Geometry check sheet. Reference: the model listing, model coordinates, mm. Face numbers are marked on the shaded views. A direction names the side the tool comes from. Coordinates: 2 decimals unless noted, no trailing zeros. Order: outer loops, then holes, each group sorted by start corner. A loop starts at its lowest first (then second) coordinate and runs counter-clockwise, first axis right, second up. Notation, with made-up numbers: (17.25, 36.25) - (43.25, 36.25) arc R26 ccw to (43.25, 75.25) - close; hole circle Ø8 at (-19, -29.75). An arc over 180 degrees is marked (long way). Return JSON: item names as keys, results as strings. Group by question number.
Item 1: Section check C-C on y = 19.5. Enter the section's corners in (x, z).
Item 2: Section check B-B on y = 10. Enter the section's corners in (x, z), then the cut area to 3 significant figures.
Item 3: Draft check along Y on the marked faces 3, 4 and 5. Enter one of: pulls with the +Y half, pulls with the -Y half, needs draft (parallel to the pull), parting line crosses it, or undercut.
Item 4: Tool access check on the marked faces 1 and 2. Record the directions out of +Z, -Z, +X, -X, +Y, -Y that give a thin tool (end or side, any length) a straight path to the whole face; none if there is none.
Item 5: Section check A-A on y = -18. Enter the section's corners in (x, z).
Item 6: Scan lines: probe 1 along Y at (x, z) = (-1.5, 2.25); probe 2 along Y at (x, z) = (-2, 2.5); probe 3 along Z at (x, y) = (0, -20.5). Record each from-to range of solid material in increasing order.
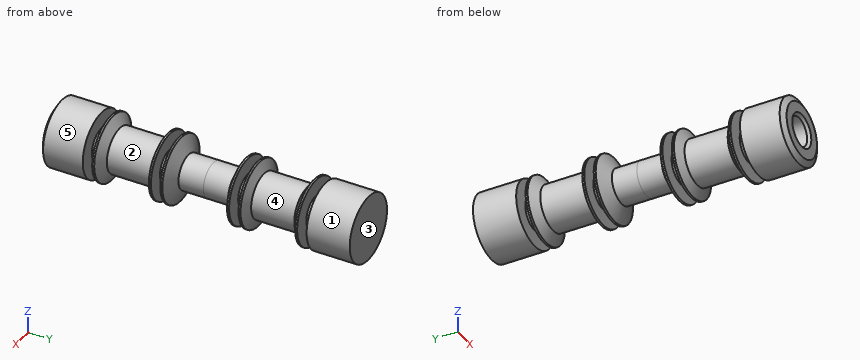
from build123d import *

# Parameters (mm, degrees)
MIDBODYS_R                           = 2.6
MIDBODY_DEPTH                        = 3.7
MIDORINGBODYS_R                      = 2.5
MIDORINGBODY_DEPTH                   = 1.4
EXTENDEDMIDBODYS_R                   = 3.35
EXTENDEDMIDBODY_DEPTH                = 6.4
ENDORINGBODYS_R                      = 2.5
ENDORINGBODY_DEPTH                   = 1.4
ENDBODY_START                        = 6.4
ENDBODYS_R                           = 4.9
ENDBODY_DEPTH                        = 6.4
F_4_2_4_2_DIAMETER_HOLE1_D           = 4.2
F_4_2_4_2_DIAMETER_HOLE1_DEPTH       = 9.4
F_4_2_4_2_DIAMETER_HOLE1_CSINK_D     = 5
F_4_2_4_2_DIAMETER_HOLE1_CSINK_ANGLE = 90
F_4_2_4_2_DIAMETER_HOLE1_TIP         = 1.2618073
CHAMFERS_OUTSIDE_W                   = 186.02
CHAMFERS_OUTSIDE_H                   = 186.02
CHAMFERS_OUTSIDE_R                   = 4
CHAMFER_2_DEPTH                      = 47.519028365
CHAMFER_2_DRAFT                      = -60


with BuildPart() as part:
    # MidBodyS → MidBody (new body)
    with BuildSketch(Plane(origin=(0, 0, 0), x_dir=(1, 0, 0), z_dir=(0, 1, 0))):
        with Locations(Location((0, 0, 0), (0, 0, 270))):
            Circle(MIDBODYS_R)
    midbody = extrude(amount=MIDBODY_DEPTH)

    # MidORingBaseS → MidORingBase (revolve)
    with BuildSketch(Plane.XY, mode=Mode.PRIVATE) as midoringbase_sk:
        Polygon((2.6, 3.7), (4.9, 4.8), (4.9, 5.1), (0, 5.1), (0, 3.7), align=None)
    midoringbase = revolve(midoringbase_sk.sketch.rotate(Axis((0, 5.1, 0), (0, -1, 0)), 180), axis=Axis((0, 5.1, 0), (0, -1, 0)))

    # MidORingBodyS → MidORingBody (add)
    with BuildSketch(Plane(origin=(0, 5.1, 0), x_dir=(1, 0, 0), z_dir=(0, 1, 0))):
        with Locations(Location((0, 0, 0), (0, 0, 180))):
            Circle(MIDORINGBODYS_R)
    midoringbody = extrude(amount=MIDORINGBODY_DEPTH)

    # MidORingTopBaseS → MidORingTopBase (revolve)
    with BuildSketch(Plane.XY, mode=Mode.PRIVATE) as midoringtopbase_sk:
        Polygon((0, 6.5), (4.9, 6.5), (4.9, 6.8), (3.35, 7.5), (0, 7.5), align=None)
    midoringtopbase = revolve(midoringtopbase_sk.sketch.rotate(Axis((0, 6.5, 0), (0, 1, 0)), 90), axis=Axis((0, 6.5, 0), (0, 1, 0)))

    # ExtendedMidBodyS → ExtendedMidBody (add)
    with BuildSketch(Plane(origin=(0, 7.5, 0), x_dir=(1, 0, 0), z_dir=(0, 1, 0))):
        with Locations(Location((0, 0, 0), (0, 0, 180))):
            Circle(EXTENDEDMIDBODYS_R)
    extendedmidbody = extrude(amount=EXTENDEDMIDBODY_DEPTH)

    # EndORingBaseS → EndORingBase (revolve)
    with BuildSketch(Plane.XY, mode=Mode.PRIVATE) as endoringbase_sk:
        Polygon((0, 15.2), (4.9, 15.2), (4.9, 14.9), (3.35, 13.9), (0, 13.9), align=None)
    endoringbase = revolve(endoringbase_sk.sketch.rotate(Axis((0, 13.9, 0), (0, 1, 0)), 90), axis=Axis((0, 13.9, 0), (0, 1, 0)))

    # EndORingBodyS → EndORingBody (add)
    with BuildSketch(Plane(origin=(0, 15.2, 0), x_dir=(1, 0, 0), z_dir=(0, 1, 0))):
        with Locations(Location((0, 0, 0), (0, 0, 180))):
            Circle(ENDORINGBODYS_R)
    endoringbody = extrude(amount=ENDORINGBODY_DEPTH)

    # EndBodyS → EndBody (add)
    with BuildSketch(Plane(origin=(0, 16.6, 0), x_dir=(1, 0, 0), z_dir=(0, 1, 0)).offset(ENDBODY_START)):
        with Locations(Location((0, 0, 0), (0, 0, 180))):
            Circle(ENDBODYS_R)
    endbody = extrude(amount=-ENDBODY_DEPTH)

    # HalfBodyVM: MidBody, MidORingBase, MidORingBody, MidORingTopBase, ExtendedMidBody, EndORingBase, EndORingBody, EndBody across plane
    add(midbody.mirror(Plane.ZX))
    add(midoringbase.mirror(Plane.ZX))
    add(midoringbody.mirror(Plane.ZX))
    add(midoringtopbase.mirror(Plane.ZX))
    add(extendedmidbody.mirror(Plane.ZX))
    add(endoringbase.mirror(Plane.ZX))
    add(endoringbody.mirror(Plane.ZX))
    add(endbody.mirror(Plane.ZX))

    # Ø4.2 (4.2) Diameter Hole1
    with Locations(Plane(origin=(0, -23, 0), x_dir=(-1, 0, 0), z_dir=(0, -1, 0))):
        with Locations((0, 0)):
            CounterSinkHole(F_4_2_4_2_DIAMETER_HOLE1_D / 2, F_4_2_4_2_DIAMETER_HOLE1_CSINK_D / 2, depth=F_4_2_4_2_DIAMETER_HOLE1_DEPTH, counter_sink_angle=F_4_2_4_2_DIAMETER_HOLE1_CSINK_ANGLE)
            with Locations((0, 0, -(F_4_2_4_2_DIAMETER_HOLE1_DEPTH + F_4_2_4_2_DIAMETER_HOLE1_TIP / 2))):  # 118° drill point
                Cone(0, F_4_2_4_2_DIAMETER_HOLE1_D / 2, F_4_2_4_2_DIAMETER_HOLE1_TIP, mode=Mode.SUBTRACT)


with BuildPart() as chamfer_2_tool:
    # ChamferS outside → Chamfer 2 (with draft: the straight prism first)
    with BuildSketch(Plane.XZ.offset(23)):
        Rectangle(CHAMFERS_OUTSIDE_W, CHAMFERS_OUTSIDE_H)
        Circle(CHAMFERS_OUTSIDE_R, mode=Mode.SUBTRACT)
    extrude(amount=-CHAMFER_2_DEPTH)
    # Chamfer 2: the draft: its side faces are tilted about the plane it starts from
    chamfer_2_sides = [chamfer_2_tool.faces().sort_by_distance(p)[0] for p in [
        (0, 0.759514182, -93.01),
        (93.01, 0.759514182, 0),
        (0, 0.759514182, 93.01),
        (-93.01, 0.759514182, 0),
        (-4, 0.759514182, 0),
    ]]
    draft(chamfer_2_sides, Plane.XZ.offset(23), CHAMFER_2_DRAFT)


with BuildPart() as part_1:
    add(part.part)

    # Chamfer 2: cut by chamfer_2_tool
    add(chamfer_2_tool.part, mode=Mode.SUBTRACT)


solid = part_1.part
Computed:
{
 "1": {"outline": "circle Ø9.8 at (0, 0)"},
 "2": {"outline": "circle Ø6.7 at (0, 0)", "area": "35.3 mm²"},
 "3": {"face 3": "pulls with the +Y half", "face 4": "undercut", "face 5": "needs draft"},
 "4": {"face 1": "+Y, -Y", "face 2": "none"},
 "5": {"outline": "circle Ø9.8 at (0, 0); hole circle Ø4.2 at (0, 0)"},
 "6": {"probe 1": "y = -23 to -16.6, -15.2 to -6.5, -5.1 to -3.75, 3.75 to 5.1, 6.5 to 15.2, 16.6 to 23", "probe 2": "y = -23 to -16.6, -15.2 to -6.5, -5.1 to -3.99, 3.99 to 5.1, 6.5 to 15.2, 16.6 to 23", "probe 3": "z = -4.9 to -2.1, 2.1 to 4.9"}
}
